Part print with two shaded views. Sizes in mm from the minimum x, y, z corner. A direction names the side the tool comes from. Coordinates: 2 decimals unless noted, no trailing zeros. Order: outer loops, then holes, each group sorted by start corner. A loop starts at its lowest first (then second) coordinate and runs counter-clockwise, first axis right, second up.
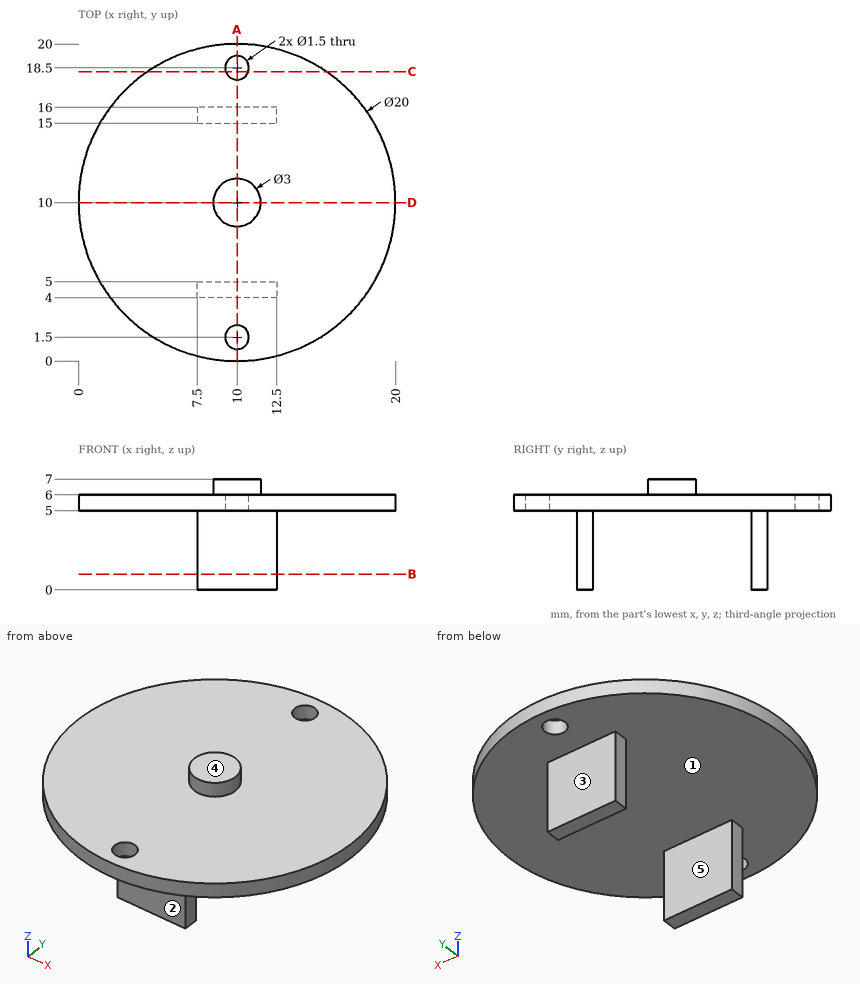
Q1. Cut at A-A on x = 10. Write the cut outline in (y, z).
Results list:
outline: (0, 5) - (0.75, 5) - (0.75, 6) - (0, 6) - close; (2.25, 5) - (4, 5) - (4, 0) - (5, 0) - (5, 5) - (15, 5) - (15, 0) - (16, 0) - (16, 5) - (17.75, 5) - (17.75, 6) - (11.5, 6) - (11.5, 7) - (8.5, 7) - (8.5, 6) - (2.25, 6) - close; (19.25, 5) - (20, 5) - (20, 6) - (19.25, 6) - close
Q2. Cut at B-B on z = 1. Write the cut outline in (x, y), and give its area (3 significant figures).
Results list:
outline: (7.5, 4) - (12.5, 4) - (12.5, 5) - (7.5, 5) - close; (7.5, 15) - (12.5, 15) - (12.5, 16) - (7.5, 16) - close
area: 10.0 mm2
Q3. Cut at D-D on y = 10. Write the cut outline in (x, z).
Results list:
outline: (0, 5) - (20, 5) - (20, 6) - (11.5, 6) - (11.5, 7) - (8.5, 7) - (8.5, 6) - (0, 6) - close
Q4. Pin check, flat tips, straight feed: pin 1 Ø4 at (x, z) = (10.5, 2) entering from -Y; pin 2 Ø4 at (x, y) = (17.5, 17) entering from -Z; pin 3 Ø1.1 at (y, z) = (4.5, 1.5) entering from -X; pin 4 Ø1.2 at (x, y) = (10, 1.5) entering from +Z. Stop position of each tip, or through.
Results list:
pin 1: stops at y = 4
pin 2: stops at z = 5
pin 3: stops at x = 7.5
pin 4: passes through
Q5. Cut at C-C on y = 18.25. Write the cut outline in (x, z).
Results list:
outline: (4.35, 5) - (9.29, 5) - (9.29, 6) - (4.35, 6) - close; (10.71, 5) - (15.65, 5) - (15.65, 6) - (10.71, 6) - close
Q6. Which spindle directions (+Z, -Z, +X, -X, +Y, -Y) get a long thin tool onto all of the face, cutting with end or side? Do the marked faces 4 and 5. Say none if no direction does.
Results list:
face 4: +Z, +X, -X, +Y, -Y
face 5: -Z, +X, -X
Q7. Wall check: line 1 along Y through (x, z) = (10, 5.65); line 2 along Z through (x, y) = (12, 6); line 3 along X through (y, z) = (15.5, 3.75). Give the ranges that are in metal, low to high.
Results list:
line 1: y = 0 to 0.75, 2.25 to 17.75, 19.25 to 20
line 2: z = 5 to 6
line 3: x = 7.5 to 12.5
Q8. Mould opens along Y. For the marked faces 1, 2 and 3 say: pulls with the +Y half, pulls with the -Y half, needs draft (parallel to the pull), parting line crosses it, or undercut.
Results list:
face 1: undercut
face 2: pulls with the -Y half
face 3: pulls with the +Y half
